The figure shows three views and two pictorial views of one solid part (mm, origin at its lowest corner). Answer the questions. A direction names the side the tool comes from. Give positions to 0.01 mm unless a question says otherwise; leave off trailing zeros. Order: outer loops, then holes, each group sorted by start corner. A loop starts at its lowest first (then second) coordinate and runs counter-clockwise, first axis right, second up. Notation, with made-up numbers: (49, -39) - (106, -39) arc R29 cw to (106, -9) - close; hole circle Ø6 at (-11.5, -30.5). An arc over 180 degrees is marked (long way). Write item = value, one per line.
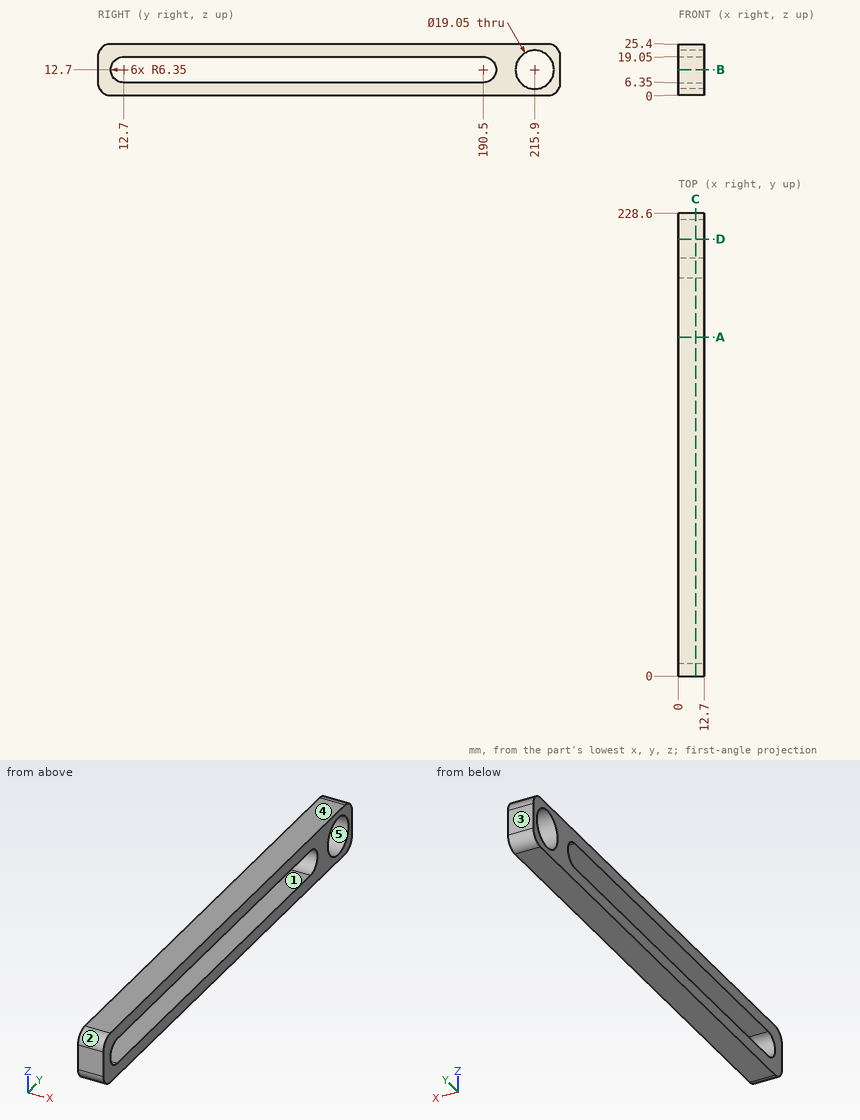
1. Straight lines are drawn through the part: L1, parallel to Z at x = 4, y = 215.9 (3 decimals); L2, parallel to Z at x = 1.5, y = 20; L3, parallel to Y at x = 3.5, z = 8. For each, find the intervals that lie inside material, in ascending order. Write a range as [from, to].
Recorded:
L1 = [0, 3.175], [22.225, 25.4]
L2 = [0, 6.35], [19.05, 25.4]
L3 = [0, 8.43], [194.77, 207.62], [224.18, 228.6]
2. Section B-B (z = 12.7) is taken. Determine the outline of the cut face in (x, y) (3 decimals), and give its area (3 significant figures).
Recorded:
outline = (0, 0) - (12.7, 0) - (12.7, 6.35) - (0, 6.35) - close; (0, 196.85) - (12.7, 196.85) - (12.7, 206.375) - (0, 206.375) - close; (0, 225.425) - (12.7, 225.425) - (12.7, 228.6) - (0, 228.6) - close
area = 242 mm^2
3. For the marked faces 1 and 2, determine the directions among +Z, -Z, +X, -X, +Y, -Y from which every point of the face is accessible in a straight line to the end or side of a thin tool.
Recorded:
face_1 = +X, -X
face_2 = +Z, +X, -X, -Y
4. Section C-C (x = 8.5) is taken. Determine the outline of the cut face in (y, z) (3 decimals), and give its area (3 significant figures).
Recorded:
outline = (0, 6.35) arc R6.35 ccw to (6.35, 0) - (222.25, 0) arc R6.35 ccw to (228.6, 6.35) - (228.6, 19.05) arc R6.35 ccw to (222.25, 25.4) - (6.35, 25.4) arc R6.35 ccw to (0, 19.05) - close; hole (12.7, 6.35) - (190.5, 6.35) arc R6.35 ccw to (190.5, 19.05) - (12.7, 19.05) arc R6.35 ccw to start; hole circle Ø19.05 at (215.9, 12.7)
area = 3,100 mm^2
5. Determine the mould class of the marked faces 3, 4 and 5 for opening direction Y: +Y half, -Y half, draft (parallel to the pull), parting line (faces both ways), or undercut.
Recorded:
face_3 = +Y half
face_4 = draft
face_5 = undercut
6. Section D-D (y = 215.9) is taken. Determine the outline of the cut face in (x, z) (3 decimals), and give its area (3 significant figures).
Recorded:
outline = (0, 0) - (12.7, 0) - (12.7, 3.175) - (0, 3.175) - close; (0, 22.225) - (12.7, 22.225) - (12.7, 25.4) - (0, 25.4) - close
area = 80.6 mm^2
7. Section A-A (y = 167.5) is taken. Determine the outline of the cut face in (x, z).
Recorded:
outline = (0, 0) - (12.7, 0) - (12.7, 6.35) - (0, 6.35) - close; (0, 19.05) - (12.7, 19.05) - (12.7, 25.4) - (0, 25.4) - close
